Build history of the part. All positions in model axes, mm. Give positions to 0.01 mm unless a question says otherwise; leave off trailing zeros. Write each loop counter-clockwise with the first axis right and the second up, starting at its lowest first coordinate (ties: lowest second). Pieces come first, ordered by that corner, then holes.
from build123d import *

# Parameters (mm, degrees)
F0_W     = 107.95
F0_H     = 12.7
F1_DEPTH = 6.35


with BuildPart() as f1:
    # F0 (on Top) → F1 (new body)
    with BuildSketch(Plane.XY):
        Polygon((-69.85, -279.4), (0, 0), (-107.95, 0), (-107.95, -279.4), align=None)
        Polygon((-107.95, 25.4), (0, 25.4), (-69.85, 304.8), (-107.95, 304.8), align=None)
        with Locations((-53.975, 19.05)):
            Rectangle(F0_W, F0_H)
        with Locations((-53.975, 6.35)):
            Rectangle(F0_W, F0_H)
    extrude(amount=F1_DEPTH)


solid = f1.part
1. Drill centre lines: line 1 along X through (y, z) = (-129.5, 3.25) (3 decimals); line 2 along X through (y, z) = (97.5, 1.5) (3 decimals). Where is each one in solid material? Low to high.
2. Mould opens along Z. For faces 1 (the face through (-67, 17, 0)), 2 (the face through (-67, 17, 6.35)), 3 (the face through (-35.414, -141.656, 3.131)) say: pulls with the +Z half, pulls with the -Z half, needs draft (parallel to the pull), parting line crosses it, or undercut.
3. Saw through at A-A on z = 3.5. Give the cut face in (x, y), plus the area to 3 significant figures.
4. Saw through at C-C on y = -124.5. Give the cut face in (x, z) (3 decimals).
5. Saw through at B-B on x = -51. Give the cut face in (y, z), plus the area to 3 significant figures.
Outcome:
1. line 1: x = -107.95 to -32.375
1. line 2: x = -107.95 to -18.025
2. face 1: pulls with the -Z half
2. face 2: pulls with the +Z half
2. face 3: needs draft
3. outline: (-107.95, -279.4) - (-69.85, -279.4) - (0, 0) - (0, 25.4) - (-69.85, 304.8) - (-107.95, 304.8) - close
3. area: 43,500 mm2
4. outline: (-107.95, 0) - (-31.125, 0) - (-31.125, 6.35) - (-107.95, 6.35) - close
5. outline: (-204, 0) - (229.4, 0) - (229.4, 6.35) - (-204, 6.35) - close
5. area: 2,750 mm2
